Source: three-view drawing plus pictorial views. Frame: mm from the lowest corner of the part. Round coordinates to 2 decimals unless told otherwise and drop trailing zeros. Write each loop counter-clockwise with the first axis right and the second up, starting at its lowest first coordinate (ties: lowest second). Pieces come first, ordered by that corner, then holes. Notation, with made-up numbers: M 41.5,-5 L 65.5,-5 A9 ccw 65.5,9 Z; hole C 84.25,67 d10. An arc over 180 degrees is marked long. Answer in a Markdown table with one row per item.
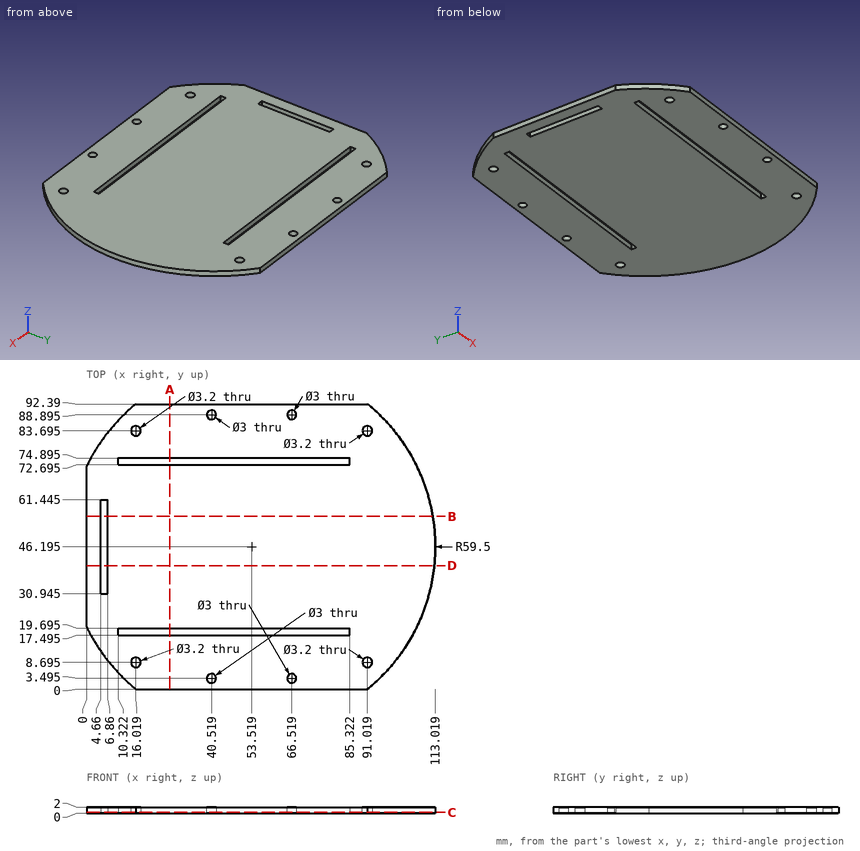
Q1. Section C-C (z = 0.3). State how many separate pieces and enclosed holes the cut face has, and give its area (3 significant figures).
Solutions:
| item | result |
|---|---|
| separate pieces | 1 |
| enclosed holes | 11 |
| area | 9,090 mm2 |
Q2. Section D-D (y = 40). Return loops of the section in (x, z) (1 decimal), and give its area (3 significant figures).
Solutions:
| item | result |
|---|---|
| outline | M 0,0 L 4.7,0 L 4.7,2 L 0,2 Z; M 6.9,0 L 112.7,0 L 112.7,2 L 6.9,2 Z |
| area | 221 mm2 |
Q3. Section B-B (y = 56). Return loops of the section in (x, z) (1 decimal), and give its area (3 significant figures).
Solutions:
| item | result |
|---|---|
| outline | M 0,0 L 4.7,0 L 4.7,2 L 0,2 Z; M 6.9,0 L 112.2,0 L 112.2,2 L 6.9,2 Z |
| area | 220 mm2 |
Q4. Contact query for flat-ended pins moving along their axis: pin 1 Ø1.8 at (x, y) = (66.52, 88.9) entering from -Z; pin 2 Ø0.6 at (y, z) = (19, 1.5) entering from -X (1 decimal); pin 3 Ø0.6 at (y, z) = (39.5, 1.5) entering from +X; pin 4 Ø1 at (y, z) = (18.5, 0.5) entering from +X. Output: stop coordinate, or through.
Solutions:
| item | result |
|---|---|
| pin 1 | passes through |
| pin 2 | stops at x = 0.4 |
| pin 3 | stops at x = 112.67 |
| pin 4 | stops at x = 106.44 |
Q5. Material intervals for probe 1 along Y at (x, z) = (43, 0.6) (1 decimal); probe 2 along X at (y, z) = (8, 0.55) (1 decimal); probe 3 along X at (y, z) = (83, 1.3), sorted ascending.
Solutions:
| item | result |
|---|---|
| probe 1 | y = 0 to 17.5, 19.7 to 72.7, 74.9 to 92.4 |
| probe 2 | x = 7.9 to 14.6, 17.5 to 89.6, 92.5 to 99.1 |
| probe 3 | x = 6.77 to 14.58, 17.46 to 89.58, 92.46 to 100.27 |
Q6. Section A-A (x = 27). Return loops of the section in (y, z) (1 decimal), and give its area (3 significant figures).
Solutions:
| item | result |
|---|---|
| outline | M 0,0 L 17.5,0 L 17.5,2 L 0,2 Z; M 19.7,0 L 72.7,0 L 72.7,2 L 19.7,2 Z; M 74.9,0 L 92.4,0 L 92.4,2 L 74.9,2 Z |
| area | 176 mm2 |
